Read the model definition and answer for the solid it produces. Units are mm, in the model's axes. A direction names the side the tool comes from. Coordinates: 2 decimals unless noted, no trailing zeros. Order: outer loops, then holes, each group sorted by start corner. A loop starts at its lowest first (then second) coordinate and runs counter-clockwise, first axis right, second up. Notation, with made-up numbers: M 75.5,3.25 L 105.5,3.25 A14 cw 105.5,28.25 Z; hole C 9.5,49.5 d10. An arc over 180 degrees is marked long. One line per question, with ' | ' between items. Start each with the question number.
1) Find section D-D, the plane z = 8.5. Write down the section's boundary in (x, y), plus the area to 3 significant figures.
2) Find section A-A, the plane y = -6.35. Write down the section's boundary in (x, z).
3) Find section C-C, the plane z = 1.25. Write down the section's boundary in (x, y).
4) Given P1, Ø3, axis at x = -14.5, z = 6.5, coming from the -Y side; P2, Ø7.5, axis at x = -4, z = 8.5, coming from the +Y side; P3, Ø0.8, axis at y = -0.5, z = 3, coming from the -X side, each flat-ended and moving along its own axis, determine where each tip first touches the part or whether it passes through.
5) Find section B-B, the plane x = -12.7. Write down the section's boundary in (y, z), plus the area to 3 significant figures.
6) Consider probe 1 along X at (y, z) = (-10.5, 6.25); probe 2 along X at (y, z) = (-6, 5); probe 3 along Y at (x, z) = (-19.05, 5.75). Determine where each line is inside the solid, lowest interval first.
7) A tool of negligible diameter and unlimited length cuts with its end or side. For faces 5 (the face through (-7.942, -10.321, 6.141)), 6 (the face through (-13, -6, 0)), 7 (the face through (-21, -1.5, 6)), 8 (the face through (-9.45, -1, 6)), 9 (the face through (-13, -6, 12.7)), from which of +Z, -Z, +X, -X, +Y, -Y can it reach the whole face along a straight path? Write none if from no direction.
8) The mould has two halves that part along Y. Classify faces 1 (the face through (-15.95, -1, 6)), 2 (the face through (-7.84, -4.99, 6.26)), 3 (the face through (-5, -1.5, 6)), 4 (the face through (-15, -7.874, 8)): +Y half, -Y half, draft (parallel to the pull), parting line (faces both ways), or undercut.
from build123d import *

# Parameters (mm, degrees)
SKETCH5_W                                       = 25.4
SKETCH5_H                                       = 12.7
BOSS_EXTRUDE2_DEPTH                             = 12.7
F_10_32_TAPPED_HOLE1_D                          = 4.0386
SKETCH6_W                                       = 9.45
SKETCH6_H                                       = 1.5
CUT_EXTRUDE1_DEPTH                              = 12.7
CBORE_FOR_10_SOCKET_HEAD_CAP_SCREW2_D           = 5.1054
CBORE_FOR_10_SOCKET_HEAD_CAP_SCREW2_CBORE_D     = 9.525
CBORE_FOR_10_SOCKET_HEAD_CAP_SCREW2_CBORE_DEPTH = 4.826


with BuildPart() as part:
    # Sketch5 → Boss-Extrude2 (new body)
    with BuildSketch(Plane.XY):
        with Locations((-12.7, -6.35)):
            Rectangle(SKETCH5_W, SKETCH5_H)
    extrude(amount=BOSS_EXTRUDE2_DEPTH)

    # #10-32 Tapped Hole1 (through all)
    with Locations(Plane.XY.offset(12.7)):
        with Locations((-19.05, -6.35)):
            f_10_32_tapped_hole1 = Hole(F_10_32_TAPPED_HOLE1_D / 2)

    # Mirror1: #10-32 Tapped Hole1 across plane
    add(f_10_32_tapped_hole1.mirror(Plane.ZY.offset(12.7)), mode=Mode.SUBTRACT)

    # Sketch6 → Cut-Extrude1 (cut)
    with BuildSketch(Plane.XY.offset(12.7)):
        with Locations((-20.675, -0.75)):
            Rectangle(SKETCH6_W, SKETCH6_H)
        with Locations((-4.725, -0.75)):
            Rectangle(SKETCH6_W, SKETCH6_H)
    extrude(amount=-CUT_EXTRUDE1_DEPTH, mode=Mode.SUBTRACT)

    # CBORE for #10 Socket Head Cap Screw2 (through all)
    with Locations(Plane(origin=(0, -12.7, 0), x_dir=(-1, 0, 0), z_dir=(0, -1, 0))):
        with Locations((12.7, -6.35)):
            CounterBoreHole(CBORE_FOR_10_SOCKET_HEAD_CAP_SCREW2_D / 2, CBORE_FOR_10_SOCKET_HEAD_CAP_SCREW2_CBORE_D / 2, CBORE_FOR_10_SOCKET_HEAD_CAP_SCREW2_CBORE_DEPTH)


solid = part.part
Report:
1) outline: M -25.4,-12.7 L -16.95,-12.7 L -16.95,-7.87 L -14.08,-7.87 L -14.08,0 L -15.95,0 L -15.95,-1.5 L -25.4,-1.5 Z; M -11.32,-7.87 L -8.45,-7.87 L -8.45,-12.7 L 0,-12.7 L 0,-1.5 L -9.45,-1.5 L -9.45,0 L -11.32,0 Z; hole C -19.05,-6.35 d4.04; hole C -6.35,-6.35 d4.04 | area: 206 mm^2
2) outline: M -25.4,0 L -21.07,0 L -21.07,12.7 L -25.4,12.7 Z; M -17.03,0 L -8.37,0 L -8.37,12.7 L -17.03,12.7 Z; M -4.33,0 L 0,0 L 0,12.7 L -4.33,12.7 Z; hole C -12.7,6.35 d5.11
3) outline: M -25.4,-12.7 L 0,-12.7 L 0,-1.5 L -9.45,-1.5 L -9.45,0 L -15.95,0 L -15.95,-1.5 L -25.4,-1.5 Z; hole C -19.05,-6.35 d4.04; hole C -6.35,-6.35 d4.04
4) P1: stops at y = -7.87 | P2: stops at y = -1.5 | P3: stops at x = -15.95
5) outline: M -12.7,0 L 0,0 L 0,3.8 L -7.87,3.8 L -7.87,1.59 L -12.7,1.59 Z; M -12.7,11.11 L -7.87,11.11 L -7.87,8.9 L 0,8.9 L 0,12.7 L -12.7,12.7 Z | area: 75.1 mm^2
6) probe 1: x = -25.4 to -17.46, -7.94 to 0 | probe 2: x = -25.4 to -21.04, -17.06 to -14.87, -10.53 to -8.34, -4.36 to 0 | probe 3: y = -12.7 to -8.37, -4.33 to -1.5
7) face 5: -Y | face 6: -Z, +X, -X, +Y, -Y | face 7: +Z, -Z, -X, +Y | face 8: +Z, -Z, +X, +Y | face 9: +Z, +X, -X, +Y, -Y
8) face 1: draft | face 2: undercut | face 3: +Y half | face 4: -Y half
